CAD build for the part. Positions are in the model's coordinates, mm. Coordinates: 2 decimals unless noted, no trailing zeros. Loops run counter-clockwise (first coordinate to the right, second up) from the corner with the lowest first, then second, coordinate; pieces in that order, holes last. Notation, with made-up numbers: (10, 73) -> (53, 73) arc R26 cw to (53, 112) -> close; hole circle Ø11 at (32.25, 45.25). An arc over 180 degrees is marked (long way). Return JSON: item names as keys, results as strings. Group by question number.
(1) Flat gauge pins, fed straight in: pin 1 Ø5 at (x, y) = (-2.5, 0) entering from -Z; pin 2 Ø4.5 at (x, y) = (0, 0) entering from +Z; pin 3 Ø1.5 at (x, z) = (1, 2) entering from +Y. Where does each tip first touch, or does it go through?
(2) Probe L1, parallel to Y at x = 0, z = 0.5; L2, parallel to Y at x = -3, z = 1.55; L3, parallel to X at y = -1.25, z = 2.3. List the from-to ranges inside material, lowest first.
(3) Saw through at C-C on z = 0.5. Write the cut outline in (x, y).
(4) Saw through at A-A on x = 0. Write the cut outline in (y, z).
(5) Saw through at D-D on z = 2.5. Write the cut outline in (x, y), then the cut area to 3 significant figures.
(6) Mould opens along Y. For faces 1 (the face through (2, 0, 0)), 2 (the face through (-1.08, -4.88, 0.86)), 3 (the face through (-1.31, -1, 0.59)) say: pulls with the +Y half, pulls with the -Y half, needs draft (parallel to the pull), parting line crosses it, or undercut.
```python
from build123d import *

# Parameters (mm, degrees)
SKETCH1_R           = 5
SKETCH1_R_2         = 1.65
BOSS_EXTRUDE1_DEPTH = 2.75
CHAMFER2_SIZE       = 1.55
FILLET1_R           = 1


with BuildPart() as part:
    # Sketch1 → Boss-Extrude1 (new body)
    with BuildSketch(Plane(origin=(0, 0, 0), x_dir=(0, 1, 0), z_dir=(0, 0, 1))):
        with Locations(Location((0, 0, 0), (0, 0, 270))):
            Circle(SKETCH1_R)
        with Locations(Location((0, 0, 0), (0, 0, 270))):
            Circle(SKETCH1_R_2, mode=Mode.SUBTRACT)
    extrude(amount=BOSS_EXTRUDE1_DEPTH)

    # Chamfer2
    chamfer2_edges = [part.edges().sort_by_distance(p)[0] for p in [
        (-1.65, 0, 2.75),
    ]]
    chamfer(chamfer2_edges, length=CHAMFER2_SIZE)

    # Fillet1
    fillet1_edges = [part.edges().sort_by_distance(p)[0] for p in [
        (-5, 0, 2.75),
    ]]
    fillet(fillet1_edges, radius=FILLET1_R)


solid = part.part
```
Geometry results:
{
 "1": {"pin 1": "z = 0", "pin 2": "z = 1.8", "pin 3": "y = 4.99"},
 "2": {"L1": "-5 to -1.65, 1.65 to 5", "L2": "-4 to 4", "L3": "-4.67 to -2.45, 2.45 to 4.67"},
 "3": {"outline": "circle Ø10 at (0, 0); hole circle Ø3.3 at (0, 0)"},
 "4": {"outline": "(-5, 0) -> (-1.65, 0) -> (-1.65, 1.2) -> (-3.2, 2.75) -> (-4, 2.75) arc R1 ccw to (-5, 1.75) -> close; (1.65, 0) -> (5, 0) -> (5, 1.75) arc R1 ccw to (4, 2.75) -> (3.2, 2.75) -> (1.65, 1.2) -> close"},
 "5": {"outline": "circle Ø9.32 at (0, 0); hole circle Ø5.9 at (0, 0)", "area": "40.9 mm²"},
 "6": {"face 1": "needs draft", "face 2": "parting line crosses it", "face 3": "undercut"}
}
